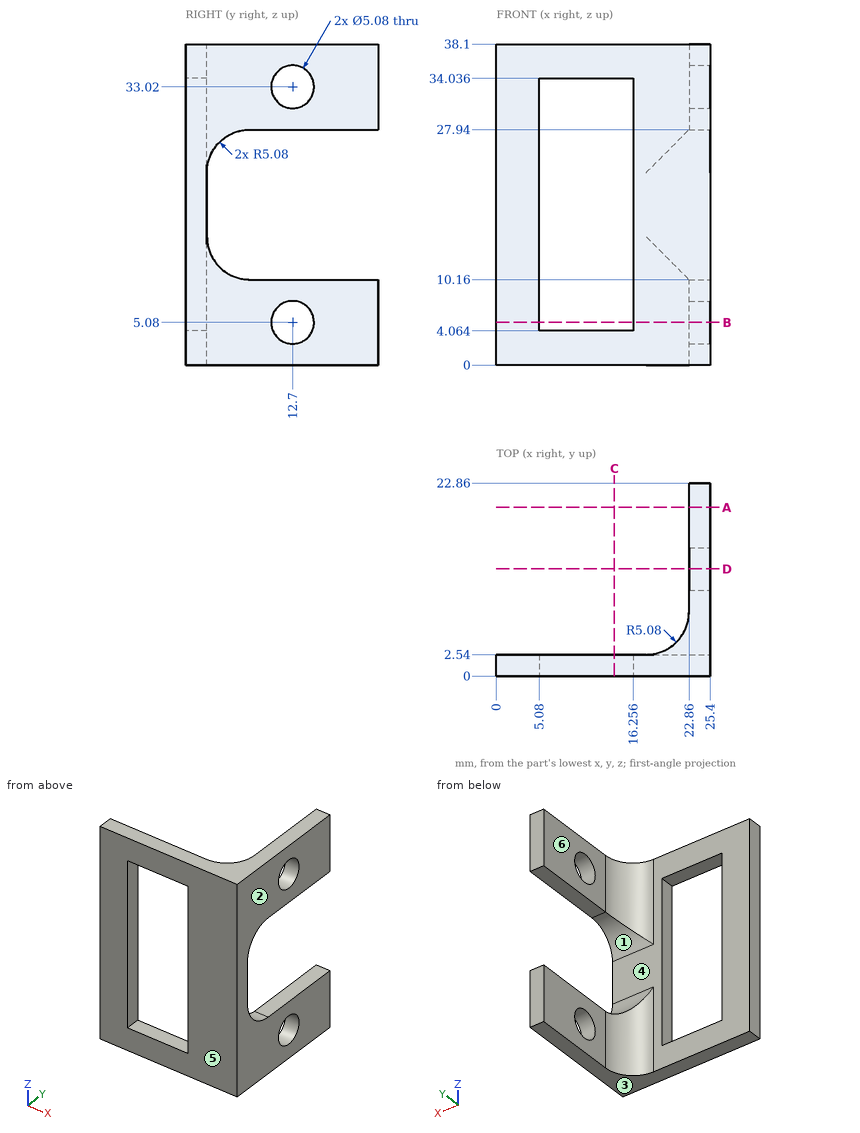
Design review of the part shown in the three views and the two pictorial views. Dimensions are in mm from the part's minimum x, y and z. A direction names the side the tool comes from. Give positions to 0.01 mm unless a question says otherwise; leave off trailing zeros. Loops run counter-clockwise (first coordinate to the right, second up) from the corner with the lowest first, then second, coordinate; pieces in that order, holes last. Notation, with made-up numbers: (-15.5, 31.5) -> (4.5, 31.5) arc R19 ccw to (4.5, 68.5) -> close; hole circle Ø4 at (-21.5, 41.5). An arc over 180 degrees is marked (long way). One line per question, with ' | ' between items.
1) The part is to be moulded in two halves that separate along Z. For the marked faces 1, 2, 3 and 4, say which applies: +Z half, -Z half, draft (parallel to the pull), parting line (faces both ways), or undercut.
Resolved:
face 1: undercut | face 2: draft | face 3: -Z half | face 4: undercut
2) We need section A-A (y = 20). Write out the cut boundary in (x, z), plus the area to 3 significant figures.
Resolved:
outline: (22.86, 0) -> (25.4, 0) -> (25.4, 10.16) -> (22.86, 10.16) -> close; (22.86, 27.94) -> (25.4, 27.94) -> (25.4, 38.1) -> (22.86, 38.1) -> close | area: 51.6 mm2
3) We need section D-D (y = 12.7). Write out the cut boundary in (x, z), plus the area to 3 significant figures.
Resolved:
outline: (22.86, 0) -> (25.4, 0) -> (25.4, 2.54) -> (22.86, 2.54) -> close; (22.86, 7.62) -> (25.4, 7.62) -> (25.4, 10.16) -> (22.86, 10.16) -> close; (22.86, 27.94) -> (25.4, 27.94) -> (25.4, 30.48) -> (22.86, 30.48) -> close; (22.86, 35.56) -> (25.4, 35.56) -> (25.4, 38.1) -> (22.86, 38.1) -> close | area: 25.8 mm2
4) We need section C-C (x = 14). Write out the cut boundary in (y, z), plus the area to 3 significant figures.
Resolved:
outline: (0, 0) -> (2.54, 0) -> (2.54, 4.06) -> (0, 4.06) -> close; (0, 34.04) -> (2.54, 34.04) -> (2.54, 38.1) -> (0, 38.1) -> close | area: 20.6 mm2
5) We need section B-B (z = 5.08). Write out the cut boundary in (x, y), plus the area to 3 significant figures.
Resolved:
outline: (0, 0) -> (5.08, 0) -> (5.08, 2.54) -> (0, 2.54) -> close; (16.26, 0) -> (25.4, 0) -> (25.4, 10.16) -> (22.86, 10.16) -> (22.86, 7.62) arc R5.08 cw to (17.78, 2.54) -> (16.26, 2.54) -> close; (22.86, 15.24) -> (25.4, 15.24) -> (25.4, 22.86) -> (22.86, 22.86) -> close | area: 80.4 mm2
6) For the marked faces 5 and 6, list the 3-axis set-ups (+Z, -Z, +X, -X, +Y, -Y) from which the entire face can be reached by the end or side of a thin tool; tool diameter is ignored.
Resolved:
face 5: +Z, -Z, +X, -X, -Y | face 6: +Z, -Z, -X, +Y
7) To check wall thickness, follow probe 1 along Z at (x, y) = (23.4, 12.7); probe 2 along Y at (x, z) = (24.55, 5.08); probe 3 along X at (y, z) = (21, 4). State the ranges of each line that lie inside material, in increasing order.
Resolved:
probe 1: z = 0 to 2.54, 7.62 to 10.16, 27.94 to 30.48, 35.56 to 38.1 | probe 2: y = 0 to 10.16, 15.24 to 22.86 | probe 3: x = 22.86 to 25.4
8) Insertion check: pin 1 Ø2 at (x, z) = (8, 31) entering from -Y; pin 2 Ø7.5 at (x, z) = (15, 16.5) entering from +Y; pin 3 Ø5 at (y, z) = (19.5, 12) entering from -X. Each pin has a flat end and moves straight along its axis. Give the tip position at first contact, or say it passes through.
Resolved:
pin 1: passes through | pin 2: stops at y = 2.57 | pin 3: stops at x = 22.86
